```python
from build123d import *

# Parameters (mm, degrees)
F0_W     = 45
F0_H     = 18
F0_W_2   = 7
F0_H_2   = 8
F1_DEPTH = 3
F2_D     = 3.5
F3_R     = 1
F5_D     = 1.5


with BuildPart() as f1:
    # F0 (on Top) → F1 (new body)
    with BuildSketch(Plane.XY):
        Rectangle(F0_W, F0_H)
        Polygon((19, 4), (19, -4), (12, -4), (12, -6.5), (-12, -6.5), (-12, -4), (-19, -4), (-19, 4), (-12, 4), (-12, 6.5), (12, 6.5), (12, 4), align=None, mode=Mode.SUBTRACT)
        with Locations((15.5, 0)):
            Rectangle(F0_W_2, F0_H_2)
        with Locations((-15.5, 0)):
            Rectangle(F0_W_2, F0_H_2)
    extrude(amount=F1_DEPTH)

    # F2 (through all)
    with Locations(Plane(origin=(0, 0, 0), x_dir=(1, 0, 0), z_dir=(0, 0, -1))):
        with Locations((-19, 4), (-19, -4), (19, -4), (19, 4)):
            Hole(F2_D / 2)

    # F3
    f3_edges = [f1.edges().sort_by_distance(p)[0] for p in [
        (22.5, 9, 1.5),
        (22.5, -9, 1.5),
        (-22.5, -9, 1.5),
        (-22.5, 9, 1.5),
    ]]
    fillet(f3_edges, radius=F3_R)

    # F5 (through all)
    with Locations(Plane.XY.offset(3)):
        with Locations((-14, 0), (14, 0)):
            Hole(F5_D / 2)


solid = f1.part
```
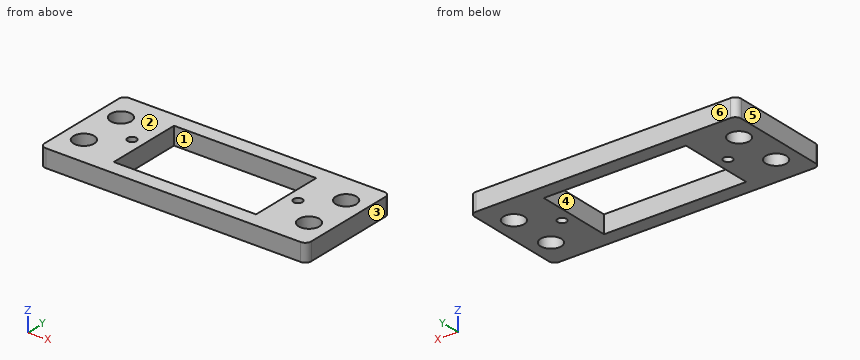
Could you check a few things on this model? Use its own coordinates, in mm. Face numbers are marked on the shaded views. A direction names the side the tool comes from. Give positions to 0.01 mm unless a question says otherwise; leave off trailing zeros. Loops run counter-clockwise (first coordinate to the right, second up) from the corner with the lowest first, then second, coordinate; pieces in that order, holes last. Notation, with made-up numbers: (-18, 76) - (-6, 76) arc R5 cw to (-6, 84) - close; hole circle Ø4 at (51.25, 54). An arc over 180 degrees is marked (long way). Use one line per item in the form item = value.
1. I want a section at C-C (x = -4). Please give me the cut outline in (y, z), and give its area (3 significant figures).
Response values:
outline = (-9, 0) - (-6.5, 0) - (-6.5, 3) - (-9, 3) - close; (6.5, 0) - (9, 0) - (9, 3) - (6.5, 3) - close
area = 15.0 mm²
2. Thinking about a two-plate mould opening in X: for the marked faces 3, 4, 5 and 6, which applies, released by +X, released by -X, zero draft, split by the parting line, or undercut?
Response values:
face_3 = released by +X
face_4 = undercut
face_5 = released by -X
face_6 = zero draft
3. I need wall thicknesses on probe 1 along Y at (x, z) = (-19, 2.05); probe 2 along X at (y, z) = (4, 1.5); probe 3 along Y at (x, z) = (-11.5, 1.1). Which ranges of each line are inside material? Lowest first, please.
Response values:
probe_1 = -9 to -5.75, -2.25 to 2.25, 5.75 to 9
probe_2 = -22.5 to -20.75, -17.25 to -12, 12 to 17.25, 20.75 to 22.5
probe_3 = -9 to -6.5, 6.5 to 9
4. I want a section at B-B (y = 4). Please give me the cut outline in (x, z).
Response values:
outline = (-22.5, 0) - (-20.75, 0) - (-20.75, 3) - (-22.5, 3) - close; (-17.25, 0) - (-12, 0) - (-12, 3) - (-17.25, 3) - close; (12, 0) - (17.25, 0) - (17.25, 3) - (12, 3) - close; (20.75, 0) - (22.5, 0) - (22.5, 3) - (20.75, 3) - close
5. I want a section at A-A (z = 1.8). Please give me the cut outline in (x, y), and give its area (3 significant figures).
Response values:
outline = (-22.5, -8) arc R1 ccw to (-21.5, -9) - (21.5, -9) arc R1 ccw to (22.5, -8) - (22.5, 8) arc R1 ccw to (21.5, 9) - (-21.5, 9) arc R1 ccw to (-22.5, 8) - close; hole circle Ø3.5 at (-19, -4); hole circle Ø3.5 at (-19, 4); hole circle Ø1.5 at (-14, 0); hole (-12, -6.5) - (12, -6.5) - (12, 6.5) - (-12, 6.5) - close; hole circle Ø1.5 at (14, 0); hole circle Ø3.5 at (19, -4); hole circle Ø3.5 at (19, 4)
area = 455 mm²
6. I want a section at D-D (x = -19). Please give me the cut outline in (y, z), and give its area (3 significant figures).
Response values:
outline = (-9, 0) - (-5.75, 0) - (-5.75, 3) - (-9, 3) - close; (-2.25, 0) - (2.25, 0) - (2.25, 3) - (-2.25, 3) - close; (5.75, 0) - (9, 0) - (9, 3) - (5.75, 3) - close
area = 33.0 mm²
7. On a 3-axis mill with a long thin cutter (end or side, diameter ignored), from which of +Z, -Z, +X, -X, +Y, -Y can I reach the whole of each face in a straight line? I mean the marked faces 1 and 2. Say none if no direction works.
Response values:
face_1 = +Z, -Z
face_2 = +Z, +X, -X, +Y, -Y
